The model under review builds one solid part; all positions refer to its coordinate system, in mm. A direction names the side the tool comes from. Round coordinates to 2 decimals unless told otherwise and drop trailing zeros. Loops run counter-clockwise (first coordinate to the right, second up) from the corner with the lowest first, then second, coordinate; pieces in that order, holes last. Notation, with made-up numbers: M 3,-18 L 49,-18 A26 cw 49,21 Z; hole C 10,56 d5. An arc over 180 degrees is marked long. Return JSON: item names as keys, results as strings. Group by question number.
Q1. Consider section C-C (z = 1.95). State the section outline as (x, y) points, and give its area (3 significant figures).
Q2. Clearance check with flat-ended pins moving along their axes: pin 1 Ø2.5 at (y, z) = (21, 1.5) entering from -X; pin 2 Ø1 at (x, z) = (8.5, 4.5) entering from +Y; pin 3 Ø0.9 at (y, z) = (108, 2) entering from -X. State where each tip first meets the part, or that it passes through.
Q3. Consider section D-D (x = 20.5). State the section outline as (y, z) points.
Q4. To check wall thickness, follow line 1 along Y through (x, z) = (16, 4.75); line 2 along Y through (x, z) = (18, 1.5); line 3 along X through (y, z) = (17, 1.8). State the ranges of each line that lie inside material, in increasing order.
Q5. For faces 5 (the face through (15, 39, 5)), 6 (the face through (9.4, 45.49, 2.46)), 7 (the face through (20.995, 42.093, 2.465)), list the 3-axis set-ups (+Z, -Z, +X, -X, +Y, -Y) from which the entire face can be reached by the end or side of a thin tool; tool diameter is ignored.
Q6. Draft analysis for pull direction X (two halves, no side actions). For faces 1 (the face through (28.642, 108, 2)), 2 (the face through (20.584, 80.506, 2.465)), 3 (the face through (12.92, 69.8, 2.46)), 4 (the face through (27.444, 87.364, 2.465)), state which applies: pulls with the +X half, pulls with the -X half, needs draft (parallel to the pull), parting line crosses it, or undercut.
Q7. Consider section A-A (x = 6). State the section outline as (y, z) points, and give its area (3 significant figures).
Q8. Consider section B-B (x = 11.5). State the section outline as (y, z) points.
from build123d import *

# Parameters (mm, degrees)
F0_R     = 1.7
F1_DEPTH = 5


with BuildPart() as f1:
    # F0 (on Top) → F1 (new body)
    with BuildSketch(Plane.XY):
        with BuildLine():
            Line((33.642043, 109.531558), (28.642043, 109.531558))
            Line((28.642043, 109.531558), (28.642043, 106.531558))
            Line((28.642043, 106.531558), (-0.036779, 65.573956))
            Line((-0.036779, 65.573956), (19.098496, 24.845081))
            Line((19.098496, 24.845081), (19.098496, 14.845081))
            Line((19.098496, 14.845081), (26.169564, 7.774013))
            Line((26.169564, 7.774013), (30.465285, 12.069734))
            ThreePointArc((30.465285, 12.069734), (32.230269, 15.466208), (31.722454, 19.260062))
            Line((31.722454, 19.260062), (9.963221, 65.573956))
            Line((9.963221, 65.573956), (15.967054, 74.148317))
            Line((15.967054, 74.148317), (25.332929, 87.043583))
            ThreePointArc((25.332929, 87.043583), (27.473238, 87.350655), (28.642043, 85.531558))
            Line((28.642043, 85.531558), (28.642043, 84.531558))
            Line((28.642043, 84.531558), (33.642043, 84.531558))
            Line((33.642043, 84.531558), (33.642043, 109.531558))
        make_face()
        with Locations((25.975157, 16.559862)):
            Circle(F0_R, mode=Mode.SUBTRACT)
        with BuildLine():
            Line((26.169564, 7.774013), (19.098496, 14.845081))
            Line((19.098496, 14.845081), (-9.185775, -13.439191))
            Line((-9.185775, -13.439191), (-6.852323, -15.772643))
            ThreePointArc((-6.852323, -15.772643), (-4.99968, -15.404129), (-3.950241, -16.974725))
            ThreePointArc((-3.950241, -16.974725), (-4.079646, -17.625286), (-4.44816, -18.176806))
            Line((-4.44816, -18.176806), (-2.114708, -20.510258))
            Line((-2.114708, -20.510258), (26.169564, 7.774013))
        make_face()
        with BuildLine():
            Line((-6.852323, -15.772643), (-9.185775, -13.439191))
            ThreePointArc((-9.185775, -13.439191), (-9.185775, -20.510258), (-2.114708, -20.510258))
            Line((-2.114708, -20.510258), (-4.44816, -18.176806))
            ThreePointArc((-4.44816, -18.176806), (-6.852323, -18.176806), (-6.852323, -15.772643))
        make_face()
    extrude(amount=F1_DEPTH)


solid = f1.part
Values:
{
 "1": {"outline": "M -9.19,-13.44 A5 ccw -2.11,-20.51 L 30.47,12.07 A6.35 ccw 31.72,19.26 L 9.96,65.57 L 15.97,74.15 L 25.33,87.04 A2 cw 28.64,85.53 L 28.64,84.53 L 33.64,84.53 L 33.64,109.53 L 28.64,109.53 L 28.64,106.53 L -0.04,65.57 L 19.1,24.85 L 19.1,14.85 Z; hole M -4.45,-18.18 A1.7 ccw -3.95,-16.97 A1.7 ccw long Z; hole C 25.98,16.56 d3.4", "area": "1,470 mm2"},
 "2": {"pin 1": "stops at x = 19.1", "pin 2": "stops at y = 78.48", "pin 3": "stops at x = 28.64"},
 "3": {"outline": "M 2.1,0 L 43.15,0 L 43.15,5 L 2.1,5 Z; M 80.39,0 L 94.9,0 L 94.9,5 L 80.39,5 Z"},
 "4": {"line 1": "y = -2.4 to 11.75, 31.44 to 52.72, 74.19 to 88.48", "line 2": "y = -0.4 to 13.75, 27.18 to 48.47, 76.95 to 91.33", "line 3": "x = 19.1 to 24.33, 27.62 to 32.31"},
 "5": {"face 5": "+Z, +X, -X, +Y, -Y", "face 6": "+Z, -Z, -X", "face 7": "+Z, -Z, +X"},
 "6": {"face 1": "pulls with the -X half", "face 2": "undercut", "face 3": "pulls with the +X half", "face 4": "undercut"},
 "7": {"outline": "M -12.4,0 L 1.75,0 L 1.75,5 L -12.4,5 Z; M 52.72,0 L 74.2,0 L 74.2,5 L 52.72,5 Z", "area": "178 mm2"},
 "8": {"outline": "M -6.9,0 L 7.25,0 L 7.25,5 L -6.9,5 Z; M 41.02,0 L 62.3,0 L 62.3,5 L 41.02,5 Z; M 67.77,0 L 82.05,0 L 82.05,5 L 67.77,5 Z"}
}
